Could you check a few things on this drawing? It's one solid part, dimensions in mm from its lowest x, y, z. Coordinates: 2 decimals unless noted, no trailing zeros. Write each loop counter-clockwise with the first axis right and the second up, starting at its lowest first coordinate (ties: lowest second). Pieces come first, ordered by that corner, then holes. Notation, with made-up numbers: (-1, 73) - (17, 73) arc R22 ccw to (17, 92) - close; hole circle Ø2 at (14, 67). An arc over 180 degrees is marked (long way). Use one line per item in the form item = value. Start each with the question number.
(1) If we section it at A-A on z = 7.5: Please give me the cut outline in (x, y).
(2) Thinking about a two-plate mould opening in X: for the marked faces 1, 2, 3 and 4, which applies, pulls with the +X half, pulls with the -X half, needs draft (parallel to the pull), parting line crosses it, or undercut?
(3) If I drill on probe 1 along Z at (x, y) = (15, 2.75); probe 2 along X at (y, z) = (0.5, 13.25); probe 3 along X at (y, z) = (4, 7), over which ranges is the centre line in solid material (lowest first)? Write a range as from..to.
(4) If we section it at B-B on x = 15: Please give me the cut outline in (y, z).
(5) If we section it at C-C on y = 2.75: Please give me the cut outline in (x, z), then the cut area to 3 significant figures.
(6) If we section it at D-D on z = 10: Please give me the cut outline in (x, y), then the cut area to 3 significant figures.
(7) For pin 1 Ø3 at (x, z) = (23, 3) entering from -Y, with a flat end and sliding along its axis, tell me the tip position at first contact or that it passes through.
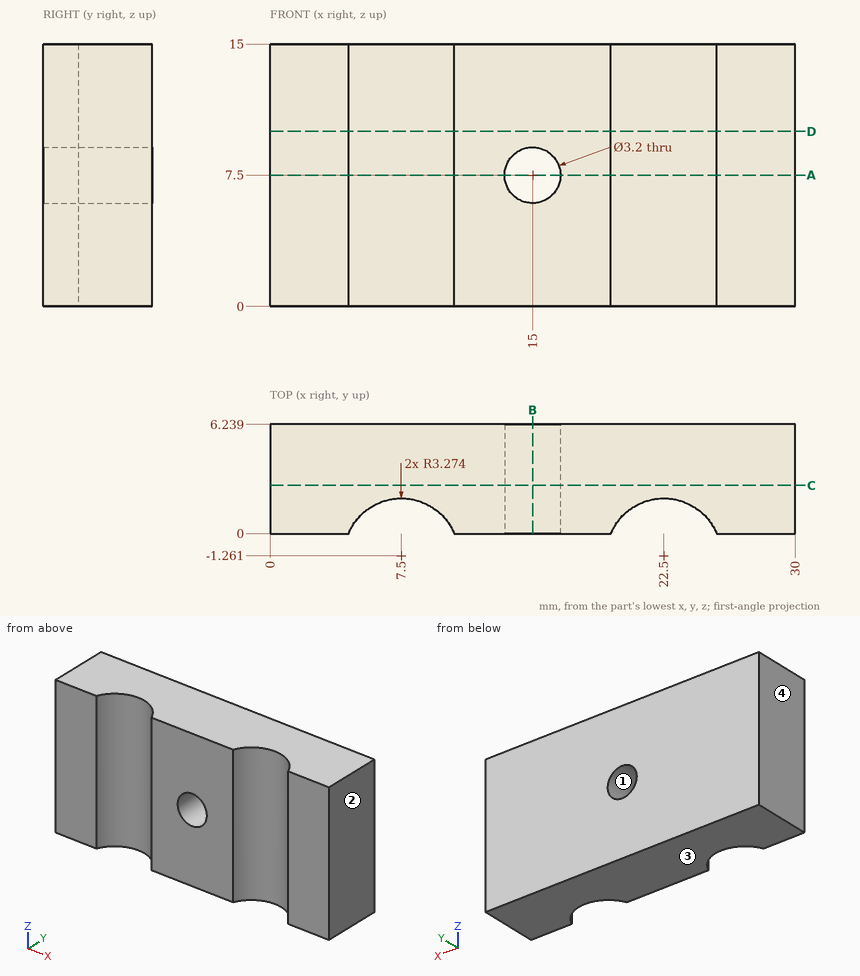
Reported:
q1.outline = (0, 0) - (4.48, 0) arc R3.27 cw to (10.52, 0) - (13.4, 0) - (13.4, 6.24) - (0, 6.24) - close; (16.6, 0) - (19.48, 0) arc R3.27 cw to (25.52, 0) - (30, 0) - (30, 6.24) - (16.6, 6.24) - close
q2.face_1 = undercut
q2.face_2 = pulls with the +X half
q2.face_3 = needs draft
q2.face_4 = pulls with the -X half
q3.probe_1 = 0..5.9, 9.1..15
q3.probe_2 = 0..4.74, 10.26..19.74, 25.26..30
q3.probe_3 = 0..13.48, 16.52..30
q4.outline = (0, 0) - (6.24, 0) - (6.24, 5.9) - (0, 5.9) - close; (0, 9.1) - (6.24, 9.1) - (6.24, 15) - (0, 15) - close
q5.outline = (0, 0) - (30, 0) - (30, 15) - (0, 15) - close; hole circle Ø3.2 at (15, 7.5)
q5.area = 442 mm2
q6.outline = (0, 0) - (4.48, 0) arc R3.27 cw to (10.52, 0) - (19.48, 0) arc R3.27 cw to (25.52, 0) - (30, 0) - (30, 6.24) - (0, 6.24) - close
q6.area = 170 mm2
q7.pin_1 = 1.33
